Check sheet for the modelled part. Datum: model origin and axes. Units: mm. A direction names the side the tool comes from. Round coordinates to 2 decimals unless told otherwise and drop trailing zeros. Write each loop counter-clockwise with the first axis right and the second up, starting at its lowest first coordinate (ties: lowest second). Pieces come first, ordered by that corner, then holes. Notation, with made-up numbers: (81.25, 18) -> (122.25, 18) arc R13 cw to (122.25, 29) -> close; hole circle Ø11 at (-9, 7.5). An arc over 180 degrees is marked (long way). One line per item, written item: value.
from build123d import *

# Parameters (mm, degrees)
CYLINDER010_R     = 4
CYLINDER010_DEPTH = 12
CYLINDER009_R     = 4
CYLINDER009_DEPTH = 12
CYLINDER006_R     = 4
CYLINDER006_DEPTH = 5
CYLINDER005_R     = 2.5
CYLINDER005_DEPTH = 5
CYLINDER003_R     = 2
CYLINDER003_DEPTH = 6
CYLINDER002_R     = 2
CYLINDER002_DEPTH = 6
BOX_W             = 10
BOX_H             = 12
BOX_DEPTH         = 80


with BuildPart() as cylinder010:
    # Cylinder010 → Cylinder010 (new body)
    with BuildSketch(Plane(origin=(10, 10, 63), x_dir=(1, 0, 0), z_dir=(0, -1, 0))):
        Circle(CYLINDER010_R)
    extrude(amount=CYLINDER010_DEPTH)


with BuildPart() as fusion005:
    # Cylinder009 → Cylinder009 (new body)
    with BuildSketch(Plane(origin=(10, 10, 47), x_dir=(1, 0, 0), z_dir=(0, -1, 0))):
        Circle(CYLINDER009_R)
    extrude(amount=CYLINDER009_DEPTH)

    # Fusion005: union Cylinder010
    add(cylinder010.part)


with BuildPart() as fusion005_1:
    # Fusion005 placement: moved
    add(fusion005.part.moved(Location((22, 2, 0))))


with BuildPart() as cylinder006:
    # Cylinder006 → Cylinder006 (new body)
    with BuildSketch(Plane(origin=(37, 5, 55), x_dir=(0, 0, -1), z_dir=(1, 0, 0))):
        Circle(CYLINDER006_R)
    extrude(amount=CYLINDER006_DEPTH)


with BuildPart() as fusion003:
    # Cylinder005 → Cylinder005 (new body)
    with BuildSketch(Plane(origin=(32, 5, 55), x_dir=(0, 0, -1), z_dir=(1, 0, 0))):
        Circle(CYLINDER005_R)
    extrude(amount=CYLINDER005_DEPTH)

    # Fusion003: union Cylinder006
    add(cylinder006.part)


with BuildPart() as fusion003_1:
    # Fusion003 placement: moved
    add(fusion003.part.moved(Location((0, 1, 0))))


with BuildPart() as cylinder003:
    # Cylinder003 → Cylinder003 (new body)
    with BuildSketch(Plane(origin=(10, 5, 40), x_dir=(0, 0, -1), z_dir=(1, 0, 0))):
        Circle(CYLINDER003_R)
    extrude(amount=CYLINDER003_DEPTH)


with BuildPart() as clipsnegative:
    # Cylinder002 → Cylinder002 (new body)
    with BuildSketch(Plane(origin=(10, 5, 70), x_dir=(0, 0, -1), z_dir=(1, 0, 0))):
        Circle(CYLINDER002_R)
    extrude(amount=CYLINDER002_DEPTH)

    # Fusion001: union Cylinder003
    add(cylinder003.part)


with BuildPart() as clipsnegative_1:
    # Fusion001 placement: moved
    add(clipsnegative.part.moved(Location((22, 1, 0))))


with BuildPart() as obj1:
    # Box → Box (new body)
    with BuildSketch(Plane(origin=(32, 0, 0), x_dir=(1, 0, 0), z_dir=(0, 0, 1))):
        with Locations((5, 6)):
            Rectangle(BOX_W, BOX_H)
    extrude(amount=BOX_DEPTH)

    # Cut: cut ClipsNegative
    add(clipsnegative_1.part, mode=Mode.SUBTRACT)

    # Cut002: cut Fusion003
    add(fusion003_1.part, mode=Mode.SUBTRACT)

    # Cut004: cut Fusion005
    add(fusion005_1.part, mode=Mode.SUBTRACT)


solid = obj1.part
Item 1: Sectioned sample at D-D on x = 40. Enter the section's corners in (y, z).
Answer:
outline: (0, 0) -> (12, 0) -> (12, 80) -> (0, 80) -> close; hole circle Ø8 at (6, 55)
Item 2: Tool access check on faces 1 (the cylindrical face through (34.465, 6.751, 52.615)), 2 (the cylindrical face through (39.465, 7.201, 51.185)), 3 (the flat face through (38, 6, 70)). Record the directions out of +Z, -Z, +X, -X, +Y, -Y that give a thin tool (end or side, any length) a straight path to the whole face; none if there is none.
Answer:
face 1: +X, -X
face 2: +X
face 3: -X
Item 3: Sectioned sample at A-A on z = 55. Enter the section's corners in (x, y), and give its area (3 significant figures).
Answer:
outline: (32, 0) -> (42, 0) -> (42, 2) -> (37, 2) -> (37, 3.5) -> (32, 3.5) -> close; (32, 8.5) -> (37, 8.5) -> (37, 10) -> (42, 10) -> (42, 12) -> (32, 12) -> close
area: 55.0 mm^2
Item 4: Sectioned sample at B-B on y = 6. Enter the section's corners in (x, z).
Answer:
outline: (32, 0) -> (42, 0) -> (42, 51) -> (37, 51) -> (37, 52.5) -> (32, 52.5) -> (32, 51) arc R4 cw to (32, 43) -> (32, 42) -> (38, 42) -> (38, 38) -> (32, 38) -> close; (32, 57.5) -> (37, 57.5) -> (37, 59) -> (42, 59) -> (42, 80) -> (32, 80) -> (32, 72) -> (38, 72) -> (38, 68) -> (32, 68) -> (32, 67) arc R4 cw to (32, 59) -> close
Item 5: Mould release check, pull along Z, two halves, no side actions. Record for faces 4 (the cylindrical face through (36, 6, 47)), 5 (the flat face through (37, 0, 39)), 6 (the flat face through (37, 6, 80)): pulls with the +Z half, pulls with the -Z half, needs draft (parallel to the pull), parting line crosses it, or undercut.
Answer:
face 4: undercut
face 5: needs draft
face 6: pulls with the +Z half
Item 6: Sectioned sample at C-C on x = 33.75. Enter the section's corners in (y, z), and give its area (3 significant figures).
Answer:
outline: (0, 0) -> (12, 0) -> (12, 43.4) -> (0, 43.4) -> close; (0, 50.6) -> (12, 50.6) -> (12, 59.4) -> (0, 59.4) -> close; (0, 66.6) -> (12, 66.6) -> (12, 80) -> (0, 80) -> close; hole circle Ø5 at (6, 55); hole circle Ø4 at (6, 40); hole circle Ø4 at (6, 70)
area: 743 mm^2
Item 7: Depth check by flat-ended pin: P1, Ø5, axis at y = 6, z = 40, coming from the -X side; P2, Ø2.5, axis at y = 7.5, z = 53, coming from the +X side; P3, Ø2, axis at y = 1, z = 49, coming from the -X side. Enter the tip coordinate at first touch or a pass-through.
Answer:
P1: stops at x = 32
P2: stops at x = 37
P3: stops at x = 34.65
Item 8: Thickness scan on line 1 (Y direction, x = 33.2, z = 55); line 2 (Y direction, x = 34, z = 53.5); line 3 (Z direction, x = 33.25, y = 10.25). Record the ranges inside material, lowest first.
Answer:
line 1: y = 0 to 3.5, 8.5 to 12
line 2: y = 0 to 4, 8 to 12
line 3: z = 0 to 43.2, 50.8 to 59.2, 66.8 to 80
